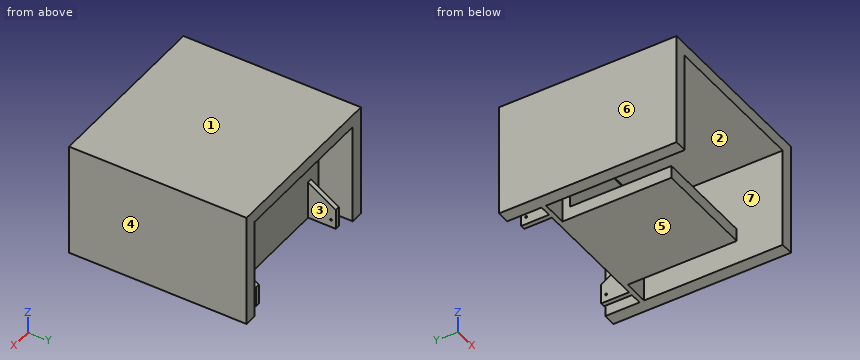
from build123d import *

# Parameters (mm, degrees)
F1_DEPTH = 700
F2_W     = 600
F2_H     = 18
F3_DEPTH = 400
F6_START = 236
F5_R     = 4
F6_DEPTH = 18
F8_DEPTH = 200


# Not quite as in the source:
# - a pattern or mirror of a feature is missing from the dataset's text; its kind, count and spacing are read off the source's solid


with BuildPart() as f1:
    # F0 (on Front) → F1 (new body)
    with BuildSketch(Plane.XZ):
        Polygon((-350, 0), (-300, 0), (-300, 400), (300, 400), (300, 0), (350, 0), (350, 450), (-350, 450), align=None)
    extrude(amount=F1_DEPTH)

    # F2 (on face) → F3 (join)
    with BuildSketch(Plane(origin=(0, 0, 400), x_dir=(1, 0, 0), z_dir=(0, 0, -1))):
        with Locations((0, 144)):
            Rectangle(F2_W, F2_H)
    extrude(amount=F3_DEPTH)

    # F5 (on Right) → F6 (join)
    with BuildSketch(Plane.YZ.offset(F6_START)):
        Polygon((-135, 150), (-135, 0), (-25, 0), (-25, 80), align=None)
        with Locations((-45, 30)):
            Circle(F5_R, mode=Mode.SUBTRACT)
    f6 = extrude(amount=F6_DEPTH)

    # F6_copies: F6 across plane
    add(f6.mirror(Plane(origin=(0, 0, 0), x_dir=(0, 0, -1), z_dir=(-1, 0, 0))))

    # F7 (on Right) → F8 (join, symmetric)
    with BuildSketch(Plane.YZ):
        Polygon((-583, 50), (-583, 0), (-153, 0), (-153, 350), (-183, 350), (-183, 50), align=None)
    extrude(amount=F8_DEPTH, both=True)


solid = f1.part
Input: part model. Units: mm. Frame: model coordinates. Face numbers are marked on the shaded views. A direction names the side the tool comes from. Give positions to 0.01 mm unless a question says otherwise; leave off trailing zeros. Order: outer loops, then holes, each group sorted by start corner. A loop starts at its lowest first (then second) coordinate and runs counter-clockwise, first axis right, second up.
Q1. Section C-C on y = -66.5. Output: boundary loops of the cut face in (x, z).
Checked values:
outline: (-350, 0) - (-300, 0) - (-300, 400) - (300, 400) - (300, 0) - (350, 0) - (350, 450) - (-350, 450) - close; (-254, 0) - (-236, 0) - (-236, 106.41) - (-254, 106.41) - close; (236, 0) - (254, 0) - (254, 106.41) - (236, 106.41) - close
Q2. Ray query, probe 1 along X at (y, z) = (-58, 46.5); probe 2 along X at (y, z) = (-522, 64); probe 3 along X at (y, z) = (-337.5, 47.5). Return the intervals inside material, ascending.
Checked values:
probe 1: x = -350 to -300, -254 to -236, 236 to 254, 300 to 350
probe 2: x = -350 to -300, 300 to 350
probe 3: x = -350 to -300, -200 to 200, 300 to 350
Q3. Section A-A on y = -377.5. Output: boundary loops of the cut face in (x, z).
Checked values:
outline: (-350, 0) - (-300, 0) - (-300, 400) - (300, 400) - (300, 0) - (350, 0) - (350, 450) - (-350, 450) - close; (-200, 0) - (200, 0) - (200, 50) - (-200, 50) - close
Q4. Section D-D on z = 166. Output: boundary loops of the cut face in (x, y).
Checked values:
outline: (-350, -700) - (-300, -700) - (-300, -153) - (-200, -153) - (-200, -183) - (200, -183) - (200, -153) - (300, -153) - (300, -700) - (350, -700) - (350, 0) - (300, 0) - (300, -135) - (-300, -135) - (-300, 0) - (-350, 0) - close
Q5. Contact query for flat-ended pins moving along their axis: pin 1 Ø15 at (x, z) = (38, 35.5) entering from -Y; pin 2 Ø5.5 at (x, z) = (247.5, 29.5) entering from +Y; pin 3 Ø12 at (x, z) = (-59.5, 290) entering from -Y. Output: stop coordinate, or through.
Checked values:
pin 1: stops at y = -583
pin 2: stops at y = -25
pin 3: stops at y = -183
Q6. Set-up query: the marked faces 1, 2 and 3. Return all of +Z, -Z, +X, -X, +Y, -Y with unobstructed straight access to the full face (end or side cutting, diameter ignored); none if empty.
Checked values:
face 1: +Z, +X, -X, +Y, -Y
face 2: -Y
face 3: -Z, +Y
Q7. Section B-B on x = 26. Output: boundary loops of the cut face in (y, z).
Checked values:
outline: (-700, 400) - (-153, 400) - (-153, 350) - (-183, 350) - (-183, 50) - (-583, 50) - (-583, 0) - (-135, 0) - (-135, 400) - (0, 400) - (0, 450) - (-700, 450) - close
Q8. Draft query along X for the marked faces 4, 5, 6 and 7. Return one class per face: +X half, -X half, draft (parallel to the pull), parting line (faces both ways), or undercut.
Checked values:
face 4: +X half
face 5: draft
face 6: -X half
face 7: undercut
